Read the model definition and answer for the solid it produces. Units are mm, in the model's axes. A direction names the side the tool comes from. Round coordinates to 2 decimals unless told otherwise and drop trailing zeros. Order: outer loops, then holes, each group sorted by start corner. A loop starts at its lowest first (then second) coordinate and runs counter-clockwise, first axis right, second up. Notation, with made-up numbers: (12.5, -8.5) - (31.5, -8.5) arc R25 cw to (31.5, 22.5) - close; hole circle Ø5 at (-18.5, 50.25). An arc over 180 degrees is marked (long way). Answer as a JSON object with one key per item and string values. Group by question number.
Q1. A cutting plane is placed at A-A on x = 13. Determine the outline of the cut face in (y, z), and give its area (4 significant figures).
Q2. A tool of negligible diameter and unlimited length cuts with its end or side. For faces 5 (the flat face through (12, 23, 15)), 6 (the flat face through (62, 23, 15)), 7 (the flat face through (37, -11, 5.041)), from which of +Z, -Z, +X, -X, +Y, -Y can it reach the whole face along a straight path? Write none if from no direction.
Q3. Consider line 1 (X direction, y = 18, z = 10.5); line 2 (Y direction, x = 13, z = 15.5); line 3 (X direction, y = 26.5, z = 16.25). Determine where each line is inside the solid, lowest interval first.
Q4. A cutting plane is placed at B-B on y = 19. Determine the outline of the cut face in (x, z), and give its area (3 significant figures).
Q5. Given pin 1 Ø3 at (x, z) = (51.5, 12) entering from +Y; pin 2 Ø5 at (x, y) = (20.5, -4) entering from -Z; pin 3 Ø4.5 at (x, y) = (33.5, -5.5) entering from -Z; pin 4 Ø12 at (x, z) = (14, 20) entering from +Y, each flat-ended and moving along its own axis, determine where each tip first touches the part or whether it passes through.
Q6. A cutting plane is placed at D-D on x = 55. Determine the outline of the cut face in (y, z), and give its area (4 significant figures).
Q7. A cutting plane is placed at C-C on z = 16. Determine the outline of the cut face in (x, y), and give its area (3 significant figures).
Q8. The mould has two halves that part along Y. Classify faces 1 (the cylindrical face through (62.582, 15.615, 8.907)), 2 (the flat face through (36, 13, 25)), 3 (the cylindrical face through (12.04, 15.69, 8.91)), 4 (the flat face through (37, -22, 13)): pulls with the +Y half, pulls with the -Y half, needs draft (parallel to the pull), parting line crosses it, or undercut.
```python
from build123d import *

# Parameters (mm, degrees)
SKETCH2_W           = 74
SKETCH2_H           = 32
BOSS_EXTRUDE1_DEPTH = 25
CUT_EXTRUDE2_DEPTH  = 25
CUT_EXTRUDE3_DEPTH  = 25
SKETCH6_R           = 5
SKETCH6_R_2         = 2.5
CUT_EXTRUDE4_DEPTH  = 33
SKETCH7_W           = 15
SKETCH7_H           = 15
BOSS_EXTRUDE2_DEPTH = 22


with BuildPart() as part:
    # Sketch2 → Boss-Extrude1 (new body)
    with BuildSketch(Plane.XY):
        with Locations((37, 16)):
            Rectangle(SKETCH2_W, SKETCH2_H)
    extrude(amount=BOSS_EXTRUDE1_DEPTH)

    # Sketch4 → Cut-Extrude2 (cut)
    with BuildSketch(Plane.ZY):
        Polygon((25, 32), (6, 32), (25, 13), align=None)
    extrude(amount=-CUT_EXTRUDE2_DEPTH, mode=Mode.SUBTRACT)

    # Sketch5 → Cut-Extrude3 (cut)
    with BuildSketch(Plane(origin=(74, 0, 0), x_dir=(0, 0, -1), z_dir=(1, 0, 0))):
        Polygon((-25, 32), (-6, 32), (-25, 13), align=None)
    extrude(amount=-CUT_EXTRUDE3_DEPTH, mode=Mode.SUBTRACT)

    # Sketch6 → Cut-Extrude4 (cut)
    with BuildSketch(Plane.XY.offset(25)):
        with Locations((36.775112994, 18.136426558)):
            Circle(SKETCH6_R)
        with Locations(Location((13, 18, 0), (0, 0, 270))):
            Circle(SKETCH6_R_2)
        with Locations(Location((61.830812036, 18, 0), (0, 0, 270))):
            Circle(SKETCH6_R_2)
    extrude(amount=-CUT_EXTRUDE4_DEPTH, mode=Mode.SUBTRACT)

    # Sketch7 → Boss-Extrude2 (add)
    with BuildSketch(Plane.XZ):
        with Locations((37, 12.541396218)):
            Rectangle(SKETCH7_W, SKETCH7_H)
    extrude(amount=BOSS_EXTRUDE2_DEPTH)


solid = part.part
```
Result set:
{
 "1": {"outline": "(0, 0) - (15.5, 0) - (15.5, 22.5) - (13, 25) - (0, 25) - close; (20.5, 0) - (32, 0) - (32, 6) - (20.5, 17.5) - close", "area": "519.5 mm²"},
 "2": {"face 5": "+Z, -X, +Y", "face 6": "+Z, +X, +Y", "face 7": "-Z, +X, -X, -Y"},
 "3": {"line 1": "x = 0 to 10.5, 15.5 to 31.78, 41.77 to 59.33, 64.33 to 74", "line 2": "y = 0 to 15.5, 20.5 to 22.5", "line 3": "x = 25 to 49"},
 "4": {"outline": "(0, 0) - (10.71, 0) - (10.71, 19) - (0, 19) - close; (15.29, 0) - (31.85, 0) - (31.85, 25) - (25, 25) - (25, 19) - (15.29, 19) - close; (41.7, 0) - (59.54, 0) - (59.54, 19) - (49, 19) - (49, 25) - (41.7, 25) - close; (64.12, 0) - (74, 0) - (74, 19) - (64.12, 19) - close", "area": "1,130 mm²"},
 "5": {"pin 1": "stops at y = 27.5", "pin 2": "passes through", "pin 3": "stops at z = 5.04", "pin 4": "stops at y = 24"},
 "6": {"outline": "(0, 0) - (32, 0) - (32, 6) - (13, 25) - (0, 25) - close", "area": "619.5 mm²"},
 "7": {"outline": "(0, 0) - (29.5, 0) - (29.5, -22) - (44.5, -22) - (44.5, 0) - (74, 0) - (74, 22) - (49, 22) - (49, 32) - (25, 32) - (25, 22) - (0, 22) - close; hole circle Ø5 at (13, 18); hole circle Ø10 at (36.78, 18.14); hole circle Ø5 at (61.83, 18)", "area": "2,080 mm²"},
 "8": {"face 1": "undercut", "face 2": "needs draft", "face 3": "undercut", "face 4": "pulls with the -Y half"}
}
